Work out the finished part from the listing and answer in its coordinate system (mm). Face numbers are marked on the shaded views. A direction names the side the tool comes from. Coordinates: 2 decimals unless noted, no trailing zeros. Order: outer loops, then holes, each group sorted by start corner. A loop starts at its lowest first (then second) coordinate and runs counter-clockwise, first axis right, second up. Notation, with made-up numbers: M 19,44 L 31,44 A16 cw 31,53 Z; hole C 12.25,2 d1. An arc over 180 degrees is marked long. Write item = value, one per line. Start each with the question number.
Q1. This flat-tipped pin is pushed along its axis until it touches: P1, Ø3.5, axis at x = 14, y = -22, coming from the -Z side. Where does it stop, or does it pass through?
Q2. Find section C-C on z = 1.5. Give the vertices of the cut face in (x, y), and give its area (3 significant figures).
Q3. Straight lines are drawn through the part: line 1 along X through (y, z) = (3, 1.45); line 2 along X through (y, z) = (2, 0.2); line 3 along Y through (x, z) = (4, 0.75). For each, find the intervals that lie inside material, in ascending order.
Q4. Find section D-D on x = -14.5. Give the vertices of the cut face in (y, z) (3 decimals).
Q5. Find section B-B on x = 7. Give the vertices of the cut face in (y, z) (3 decimals).
Q6. A tool of negligible diameter and unlimited length cuts with its end or side. For the marked faces 3, 4 and 5, from which of +Z, -Z, +X, -X, +Y, -Y can it reach the whole face along a straight path? Write none if from no direction.
Q7. Determine the mould class of the marked faces 1 and 2 for opening direction Y: released by +Y, released by -Y, zero draft, split by the parting line, or undercut.
Q8. Find section A-A on y = 0. Give the vertices of the cut face in (x, z) (3 decimals), and give its area (3 significant figures).
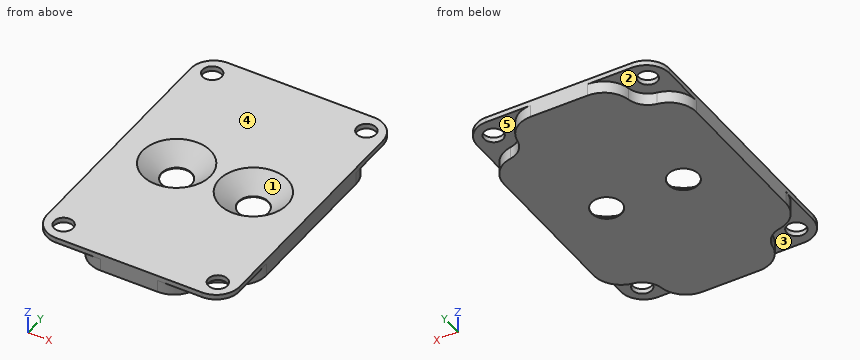
```python
from build123d import *

# Parameters (mm, degrees)
F0_R       = 1.75
F0_R_2     = 2.75
F1_DEPTH   = 3.175
F2_SIZE2   = 3.4511052217
F2_SIZE    = 3
F2_2_SIZE2 = 3.4511052217
F2_2_SIZE  = 3
F3_R       = 4
F4_DEPTH   = 2.25
F5_R       = 5


with BuildPart() as f1:
    # F0 (on Top) → F1 (new body)
    with BuildSketch(Plane.XY):
        with BuildLine():
            ThreePointArc((17.569226806, 21.6505549061), (16.324430626, 24.6557587262), (13.319226806, 25.9005549061))
            Line((13.319226806, 25.9005549061), (-13.319226806, 25.9005549061))
            ThreePointArc((-13.319226806, 25.9005549061), (-16.324430626, 24.6557587262), (-17.569226806, 21.6505549061))
            Line((-17.569226806, 21.6505549061), (-17.569226806, -21.6505549061))
            ThreePointArc((-17.569226806, -21.6505549061), (-16.324430626, -24.6557587262), (-13.319226806, -25.9005549061))
            Line((-13.319226806, -25.9005549061), (13.319226806, -25.9005549061))
            ThreePointArc((13.319226806, -25.9005549061), (16.324430626, -24.6557587262), (17.569226806, -21.6505549061))
            Line((17.569226806, -21.6505549061), (17.569226806, 21.6505549061))
        make_face()
        with Locations((-14.069226806, -22.4005549061)):
            Circle(F0_R, mode=Mode.SUBTRACT)
        with Locations((14.069226806, -22.4005549061)):
            Circle(F0_R, mode=Mode.SUBTRACT)
        with Locations((-7, 0)):
            Circle(F0_R_2, mode=Mode.SUBTRACT)
        with Locations((-14.069226806, 22.4005549061)):
            Circle(F0_R, mode=Mode.SUBTRACT)
        with Locations((7, 0)):
            Circle(F0_R_2, mode=Mode.SUBTRACT)
        with Locations((14.069226806, 22.4005549061)):
            Circle(F0_R, mode=Mode.SUBTRACT)
    extrude(amount=F1_DEPTH)

    # F2
    f2_edges = [f1.edges().sort_by_distance(p)[0] for p in [
        (-9.75, 0, 3.175),
    ]]
    f2_side = f1.faces().sort_by_distance((-9.75, 0, 1.5875))[0]
    chamfer(f2_edges, length=F2_SIZE, length2=F2_SIZE2, reference=f2_side)

    # F2#2
    f2_2_edges = [f1.edges().sort_by_distance(p)[0] for p in [
        (4.25, 0, 3.175),
    ]]
    f2_2_side = f1.faces().sort_by_distance((4.25, 0, 1.5875))[0]
    chamfer(f2_2_edges, length=F2_2_SIZE, length2=F2_2_SIZE2, reference=f2_2_side)

    # F3 (on face) → F4 (cut)
    with BuildSketch(Plane(origin=(0, 0, 0), x_dir=(1, 0, 0), z_dir=(0, 0, -1))):
        with Locations((-14.069226806, 22.4005549061)):
            Circle(F3_R)
        with Locations((14.069226806, 22.4005549061)):
            Circle(F3_R)
        with Locations((-14.069226806, -22.4005549061)):
            Circle(F3_R)
        with Locations((14.069226806, -22.4005549061)):
            Circle(F3_R)
    extrude(amount=-F4_DEPTH, mode=Mode.SUBTRACT)

    # F5
    f5_edges = [f1.edges().sort_by_distance(p)[0] for p in [
        (-12.132735, -25.900555, 1.125),
        (-17.569227, -20.464063, 1.125),
        (12.132735, -25.900555, 1.125),
        (17.569227, -20.464063, 1.125),
        (-17.569227, 20.464063, 1.125),
        (-12.132735, 25.900555, 1.125),
        (12.132735, 25.900555, 1.125),
        (17.569227, 20.464063, 1.125),
    ]]
    fillet(f5_edges, radius=F5_R)


solid = f1.part
```
Findings below:
q1.P1 = 2.25
q2.outline = M -17.57,-13.53 A5 ccw -13.4,-18.46 A4 cw -10.13,-21.73 A5 ccw -5.2,-25.9 L 5.2,-25.9 A5 ccw 10.13,-21.73 A4 cw 13.4,-18.46 A5 ccw 17.57,-13.53 L 17.57,13.53 A5 ccw 13.4,18.46 A4 cw 10.13,21.73 A5 ccw 5.2,25.9 L -5.2,25.9 A5 ccw -10.13,21.73 A4 cw -13.4,18.46 A5 ccw -17.57,13.53 Z; hole C -7,0 d8.55; hole C 7,0 d8.55
q2.area = 1,460 mm^2
q3.line_1 = -17.57 to -9.96, -4.04 to 4.04, 9.96 to 17.57
q3.line_2 = -17.57 to -8.93, -5.07 to 5.07, 8.93 to 17.57
q3.line_3 = -25.9 to -1.62, 1.62 to 25.9
q4.outline = M -25.733,2.25 L -24.097,2.25 L -24.097,3.175 L -25.733,3.175 Z; M -20.704,2.25 L -18.139,2.25 L -18.139,0 L 18.139,0 L 18.139,2.25 L 20.704,2.25 L 20.704,3.175 L -20.704,3.175 Z; M 24.097,2.25 L 25.733,2.25 L 25.733,3.175 L 24.097,3.175 Z
q5.outline = M -25.901,2.25 L -25.563,2.25 L -25.563,0 L -2.75,0 L -2.75,0.175 L -6.201,3.175 L -25.901,3.175 Z; M 2.75,0 L 25.563,0 L 25.563,2.25 L 25.901,2.25 L 25.901,3.175 L 6.201,3.175 L 2.75,0.175 Z
q6.face_3 = -Z, -X, -Y
q6.face_4 = +Z, +X, -X, +Y, -Y
q6.face_5 = -Z, +X, +Y
q7.face_1 = undercut
q7.face_2 = zero draft
q8.outline = M -17.569,0 L -9.75,0 L -9.75,0.175 L -13.201,3.175 L -17.569,3.175 Z; M -4.25,0 L 4.25,0 L 4.25,0.175 L 0.799,3.175 L -0.799,3.175 L -4.25,0.175 Z; M 9.75,0 L 17.569,0 L 17.569,3.175 L 13.201,3.175 L 9.75,0.175 Z
q8.area = 55.9 mm^2
